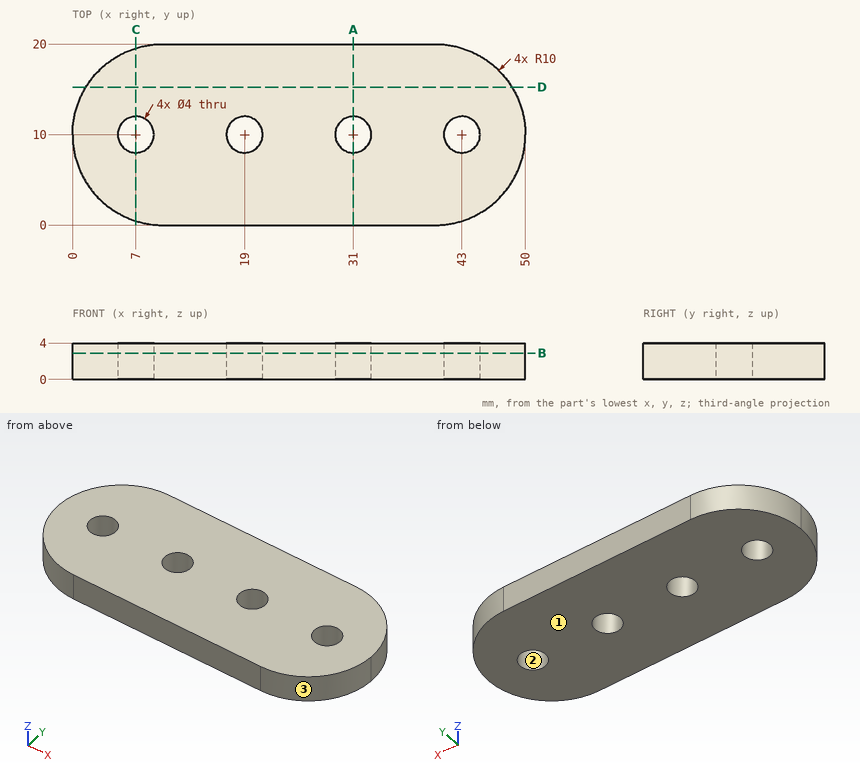
Geometry check sheet. Reference: drawing and pictorial views, mm from the part's lowest x, y, z. Round coordinates to 2 decimals unless told otherwise and drop trailing zeros. Order: outer loops, then holes, each group sorted by start corner. A loop starts at its lowest first (then second) coordinate and runs counter-clockwise, first axis right, second up.
Q1. Cross-section at A-A, the plane x = 31. Enter the section's corners in (y, z).
Filled sheet:
outline: (0, 0) - (8, 0) - (8, 4) - (0, 4) - close; (12, 0) - (20, 0) - (20, 4) - (12, 4) - close
Q2. Draft check along Y on the marked faces 1, 2 and 3. Enter one of: pulls with the +Y half, pulls with the -Y half, needs draft (parallel to the pull), parting line crosses it, or undercut.
Filled sheet:
face 1: needs draft
face 2: undercut
face 3: pulls with the -Y half
Q3. Cross-section at B-B, the plane z = 2.9. Give the number of separate pieces and of enclosed holes in the cut face, plus the area to 3 significant figures.
Filled sheet:
separate pieces: 1
enclosed holes: 4
area: 864 mm2
Q4. Cross-section at D-D, the plane y = 15.25. Enter the section's corners in (x, z).
Filled sheet:
outline: (1.49, 0) - (48.51, 0) - (48.51, 4) - (1.49, 4) - close
Q5. Depth check by flat-ended pin: P1, Ø5, axis at x = 19, y = 10, coming from the -Z side; P2, Ø3.5, axis at x = 31, y = 10, coming from the +Z side. Enter the tip coordinate at first touch or a pass-through.
Filled sheet:
P1: stops at z = 0
P2: passes through
Q6. Scan lines: L1, parallel to Y at x = 31, z = 2.5; L2, parallel to X at y = 8.5, z = 3.3; L3, parallel to Y at x = 42, z = 2.1. Record each from-to range of solid material in increasing order.
Filled sheet:
L1: y = 0 to 8, 12 to 20
L2: x = 0.11 to 5.68, 8.32 to 17.68, 20.32 to 29.68, 32.32 to 41.68, 44.32 to 49.89
L3: y = 0.2 to 8.27, 11.73 to 19.8
Q7. Cross-section at C-C, the plane x = 7. Enter the section's corners in (y, z), plus the area to 3 significant figures.
Filled sheet:
outline: (0.46, 0) - (8, 0) - (8, 4) - (0.46, 4) - close; (12, 0) - (19.54, 0) - (19.54, 4) - (12, 4) - close
area: 60.3 mm2
